Input: part model. Units: mm. Frame: model coordinates. Face numbers are marked on the shaded views. A direction names the side the tool comes from. Round coordinates to 2 decimals unless told otherwise and drop trailing zeros. Order: outer loops, then holes, each group sorted by start corner. A loop starts at its lowest first (then second) coordinate and runs counter-clockwise, first axis right, second up. Notation, with made-up numbers: (83, -10) - (141, -10) arc R27 cw to (141, 28) - close; hole circle Ø6 at (43, 40.25). An arc over 180 degrees is marked (long way). One line per item, written item: value. Start each with the question number.
from build123d import *

# Parameters (mm, degrees)
BOSS_EXTRUDE1_DEPTH = 20


with BuildPart() as part:
    # Sketch1 → Boss-Extrude1 (new body)
    with BuildSketch(Plane(origin=(0, 0, 0), x_dir=(1, 0, 0), z_dir=(0, 1, 0))):
        Polygon((0, 125), (0, -125), (86.602540378, -75), (86.602540378, 75), align=None)
        Polygon((20, -85), (20, -25), (71.961524227, -55), align=None, mode=Mode.SUBTRACT)
        Polygon((20, 25), (20, 85), (71.961524227, 55), align=None, mode=Mode.SUBTRACT)
        Polygon((20, 0), (71.961524227, 30), (71.961524227, -30), align=None, mode=Mode.SUBTRACT)
    extrude(amount=BOSS_EXTRUDE1_DEPTH)


solid = part.part
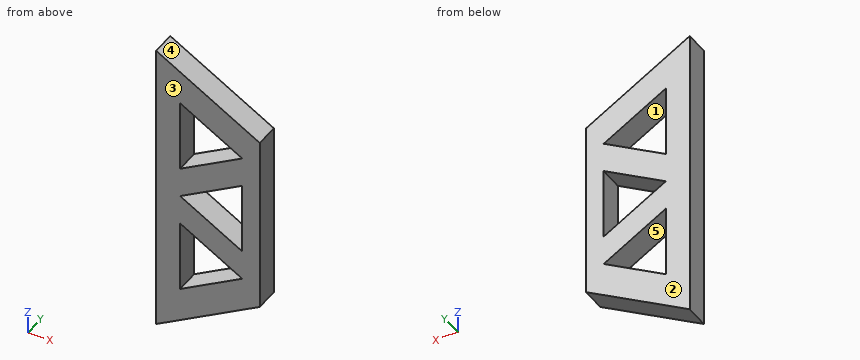
Item 1: Section query A-A on y = 3. Return loops of the section in (x, z).
Item 2: First-contact query: pin 1 Ø1.5 at (x, y) = (63, 9.5) entering from +Z; pin 2 Ø12 at (x, y) = (34.5, 6.5) entering from +Z; pin 3 Ø3 at (x, y) = (36, 15.5) entering from +Z. Flat tips, straight axial feed; report the tip coordinate or a pass-through.
Item 3: Pull-direction query (Z, two-part tool) for the marked faces 3, 4 and 5; classes: released by +Z, released by -Z, zero draft, split by the parting line, or undercut.
Item 4: Line query: L1, parallel to Z at x = 41, y = 10; L2, parallel to Z at x = 71, y = 12.5; L3, parallel to X at y = 19, z = 25.5. Output: solid intervals per line, ascending.
Item 5: Reachability of the marked faces 1 and 2 from +Z, -Z, +X, -X, +Y, -Y: full face, straight path, thin tool, end or side. Return the list, or none.
Item 6: Section query C-C on x = 48. Return loops of the section in (y, z), and give its area (3 significant figures).
Item 7: Section query D-D on z = 95.5. Return loops of the section in (x, y), and give its area (3 significant figures).
Item 8: Section query B-B on z = -79. Return loops of the section in (x, y), and give its area (3 significant figures).
Geometry results:
1. outline: (0, -125) - (86.6, -75) - (86.6, 75) - (0, 125) - close; hole (20, -85) - (71.96, -55) - (20, -25) - close; hole (20, 0) - (71.96, -30) - (71.96, 30) - close; hole (20, 25) - (71.96, 55) - (20, 85) - close
2. pin 1: stops at z = 89.06
2. pin 2: stops at z = 108.55
2. pin 3: stops at z = 105.08
3. face 3: zero draft
3. face 4: released by +Z
3. face 5: undercut
4. L1: z = -101.33 to -72.88, -37.12 to -12.12, 12.12 to 37.12, 72.88 to 101.33
4. L2: z = -84.01 to -55.56, -54.44 to -29.44, 29.44 to 54.44, 55.56 to 84.01
4. L3: x = 0 to 20, 20.87 to 64.17, 71.96 to 86.6
5. face 1: +Y, -Y
5. face 2: +Z, -Z, +X, -X, +Y
6. outline: (0, -97.29) - (20, -97.29) - (20, -68.83) - (0, -68.83) - close; (0, -41.17) - (20, -41.17) - (20, -16.17) - (0, -16.17) - close; (0, 16.17) - (20, 16.17) - (20, 41.17) - (0, 41.17) - close; (0, 68.83) - (20, 68.83) - (20, 97.29) - (0, 97.29) - close
6. area: 2,140 mm^2
7. outline: (0, 0) - (51.1, 0) - (51.1, 20) - (0, 20) - close
7. area: 1,020 mm^2
8. outline: (0, 0) - (20, 0) - (20, 20) - (0, 20) - close; (30.39, 0) - (79.67, 0) - (79.67, 20) - (30.39, 20) - close
8. area: 1,390 mm^2
